from build123d import *

# Parameters (mm, degrees)
BASE_START                 = 0.7
TOP_PROFILE_W              = 8.7
TOP_PROFILE_H              = 4.4
BASE_DEPTH                 = 4
BASE_START_2               = -2.2
BASE_EXTRUDE_DEPTH         = 4.4
BOTTOM_START               = 2.2
FRONT_PROFILE_4_W          = 4.7
FRONT_PROFILE_4_H          = 0.65
BOTTOM_FRONT_CUTOUT_DEPTH  = 0.2
BOTTOM_START_2             = -2.2
FRONT_PROFILE_5_W          = 4.7
FRONT_PROFILE_5_H          = 0.65
BOTTOM_REAR_CUTOUT_DEPTH   = 0.2
SWITCH_START               = 2.2
FRONT_PROFILE_6_W          = 4.15
FRONT_PROFILE_6_H          = 2.1
FRONT_PROFILE_6_W_2        = 2
FRONT_PROFILE_6_H_2        = 2
SWITCH_INSET_DEPTH         = 0.2
UNDERCUT_NOTCH_DEPTH       = 7.771447408
UNDERCUT_NOTCH_DEPTH_BACK  = 7.771447408
LEVER_DEPTH                = 8
LEVER_DEPTH_BACK           = 2.2
LEVER_START                = 2.2
FRONT_PROFILE_7_W          = 2
FRONT_PROFILE_7_H          = 2
RIGHT_START                = 3.95
RIGHT_PIN_DEPTH            = 0.4
LEFT_START                 = -4.35
LEFT_PIN_DEPTH             = 0.4
ELECTRICAL_PINS_DEPTH      = 4.7
ELECTRICAL_PINS_DEPTH_BACK = 2.6
PINS_R                     = 0.25
LEVER_NOTCH_DEPTH          = 13.043774325
LEVER_NOTCH_DEPTH_BACK     = 13.043774325
TOP_FILLET_R               = 0.25
PIN_FILLET_R               = 0.25


with BuildPart() as part:
    # Top Profile → Base (new body)
    with BuildSketch(Plane(origin=(0, 0, 0), x_dir=(1, 0, 0), z_dir=(0, 1, 0)).offset(BASE_START)):
        Rectangle(TOP_PROFILE_W, TOP_PROFILE_H)
    extrude(amount=BASE_DEPTH)

    # Front Profile → Base Extrude (add)
    with BuildSketch(Plane.XY.offset(BASE_START_2)):
        with BuildLine():
            Line((4.35, 0.7), (4.35, 4.7))
            Line((4.35, 4.7), (-4.35, 4.7))
            Line((-4.35, 4.7), (-4.35, 0.7))
            Line((-4.35, 0.7), (-3.35, 0.7))
            Line((-3.35, 0.7), (-3.35, 0.25))
            ThreePointArc((-3.35, 0.25), (-3.276776695, 0.073223305), (-3.1, 0))
            Line((-3.1, 0), (-2.6, 0))
            ThreePointArc((-2.6, 0), (-2.423223305, 0.073223305), (-2.35, 0.25))
            Line((-2.35, 0.25), (-2.35, 0.7))
            Line((-2.35, 0.7), (-2.35, 1.35))
            Line((-2.35, 1.35), (2.35, 1.35))
            Line((2.35, 1.35), (2.35, 0.7))
            Line((2.35, 0.7), (2.35, 0.25))
            ThreePointArc((2.35, 0.25), (2.423223305, 0.073223305), (2.6, 0))
            Line((2.6, 0), (3.1, 0))
            ThreePointArc((3.1, 0), (3.276776695, 0.073223305), (3.35, 0.25))
            Line((3.35, 0.25), (3.35, 0.7))
            Line((3.35, 0.7), (4.35, 0.7))
        make_face()
    extrude(amount=BASE_EXTRUDE_DEPTH)

    # Front Profile<4> → Bottom Front Cutout (cut)
    with BuildSketch(Plane.XY.offset(BOTTOM_START)):
        with Locations((0, 1.025)):
            Rectangle(FRONT_PROFILE_4_W, FRONT_PROFILE_4_H)
    extrude(amount=-BOTTOM_FRONT_CUTOUT_DEPTH, mode=Mode.SUBTRACT)

    # Front Profile<5> → Bottom Rear Cutout (cut)
    with BuildSketch(Plane.XY.offset(BOTTOM_START_2)):
        with Locations((0, 1.025)):
            Rectangle(FRONT_PROFILE_5_W, FRONT_PROFILE_5_H)
    extrude(amount=BOTTOM_REAR_CUTOUT_DEPTH, mode=Mode.SUBTRACT)

    # Front Profile<6> → Switch Inset (cut)
    # profile 1 of 2: a face of its own
    with BuildSketch(Plane.XY.offset(SWITCH_START)):
        with Locations((0, 2.55)):
            Rectangle(FRONT_PROFILE_6_W, FRONT_PROFILE_6_H)
        with Locations((-1, 2.55)):
            Rectangle(FRONT_PROFILE_6_W_2, FRONT_PROFILE_6_H_2, mode=Mode.SUBTRACT)
    # profile 2 of 2: a face of its own
    with BuildSketch(Plane.XY.offset(SWITCH_START)):
        with Locations((-1, 2.55)):
            Rectangle(FRONT_PROFILE_6_W_2, FRONT_PROFILE_6_H_2)
    extrude(amount=-SWITCH_INSET_DEPTH, mode=Mode.SUBTRACT)

    # Side Profile → Undercut Notch (cut, two sides: drawn at the far end of the back side and taken through both)
    with BuildSketch(Plane(origin=(0, 0, 0), x_dir=(0, 0, -1), z_dir=(1, 0, 0)).offset(-UNDERCUT_NOTCH_DEPTH_BACK)):
        with BuildLine():
            ThreePointArc((-1.2, 0), (-0.8, 0.4), (-0.4, 0))
            Line((-0.4, 0), (-1.2, 0))
        make_face()
        with BuildLine():
            ThreePointArc((0.4, 0), (0.8, 0.4), (1.2, 0))
            Line((1.2, 0), (0.4, 0))
        make_face()
        with BuildLine():
            ThreePointArc((-0.8, 0.4), (-0.517157288, 0.282842712), (-0.4, 0))
            Line((-0.4, 0), (0.4, 0))
            ThreePointArc((0.4, 0), (0.517157288, 0.282842712), (0.8, 0.4))
            Line((0.8, 0.4), (-0.8, 0.4))
        make_face()
    extrude(amount=UNDERCUT_NOTCH_DEPTH + UNDERCUT_NOTCH_DEPTH_BACK, mode=Mode.SUBTRACT)

    # Front Profile<7> → Lever (add, two sides: drawn at the far end of the back side and taken through both)
    with BuildSketch(Plane.XY.offset(LEVER_START - LEVER_DEPTH_BACK)):
        with Locations((-1, 2.55)):
            Rectangle(FRONT_PROFILE_7_W, FRONT_PROFILE_7_H)
    extrude(amount=LEVER_DEPTH + LEVER_DEPTH_BACK)

    # Side Profile<5> → Right Pin (add)
    with BuildSketch(Plane(origin=(0, 0, 0), x_dir=(0, 0, -1), z_dir=(1, 0, 0)).offset(RIGHT_START)):
        Polygon((-0.4, 0), (0.4, 0), (0.6, -1.25), (0.15, -2.5), (-0.15, -2.5), (-0.6, -1.25), align=None)
        with BuildLine():
            ThreePointArc((-0.8, 0.4), (-0.517157288, 0.282842712), (-0.4, 0))
            Line((-0.4, 0), (0.4, 0))
            ThreePointArc((0.4, 0), (0.517157288, 0.282842712), (0.8, 0.4))
            Line((0.8, 0.4), (-0.8, 0.4))
        make_face()
        with BuildLine():
            Line((2.2, 4.7), (-2.2, 4.7))
            Line((-2.2, 4.7), (-2.2, 0.7))
            Line((-2.2, 0.7), (-2.2, 0))
            Line((-2.2, 0), (-1.2, 0))
            ThreePointArc((-1.2, 0), (-1.082842712, 0.282842712), (-0.8, 0.4))
            Line((-0.8, 0.4), (0.8, 0.4))
            ThreePointArc((0.8, 0.4), (1.082842712, 0.282842712), (1.2, 0))
            Line((1.2, 0), (2.2, 0))
            Line((2.2, 0), (2.2, 0.7))
            Line((2.2, 0.7), (2.2, 4.7))
        make_face()
    extrude(amount=RIGHT_PIN_DEPTH)

    # Side Profile<6> → Left Pin (add)
    with BuildSketch(Plane(origin=(0, 0, 0), x_dir=(0, 0, -1), z_dir=(1, 0, 0)).offset(LEFT_START)):
        Polygon((-0.4, 0), (0.4, 0), (0.6, -1.25), (0.15, -2.5), (-0.15, -2.5), (-0.6, -1.25), align=None)
        with BuildLine():
            ThreePointArc((-0.8, 0.4), (-0.517157288, 0.282842712), (-0.4, 0))
            Line((-0.4, 0), (0.4, 0))
            ThreePointArc((0.4, 0), (0.517157288, 0.282842712), (0.8, 0.4))
            Line((0.8, 0.4), (-0.8, 0.4))
        make_face()
        with BuildLine():
            Line((2.2, 4.7), (-2.2, 4.7))
            Line((-2.2, 4.7), (-2.2, 0.7))
            Line((-2.2, 0.7), (-2.2, 0))
            Line((-2.2, 0), (-1.2, 0))
            ThreePointArc((-1.2, 0), (-1.082842712, 0.282842712), (-0.8, 0.4))
            Line((-0.8, 0.4), (0.8, 0.4))
            ThreePointArc((0.8, 0.4), (1.082842712, 0.282842712), (1.2, 0))
            Line((1.2, 0), (2.2, 0))
            Line((2.2, 0), (2.2, 0.7))
            Line((2.2, 0.7), (2.2, 4.7))
        make_face()
    extrude(amount=LEFT_PIN_DEPTH)

    # Pins → Electrical Pins (add, two sides: drawn at the far end of the back side and taken through both)
    with BuildSketch(Plane(origin=(0, 0, 0), x_dir=(1, 0, 0), z_dir=(0, 1, 0)).offset(-ELECTRICAL_PINS_DEPTH_BACK)):
        with Locations(Location((-2, 0, 0), (0, 0, 270))):
            Circle(PINS_R)
        with Locations(Location((0, 0, 0), (0, 0, 270))):
            Circle(PINS_R)
        with Locations(Location((2, 0, 0), (0, 0, 270))):
            Circle(PINS_R)
    extrude(amount=ELECTRICAL_PINS_DEPTH + ELECTRICAL_PINS_DEPTH_BACK)

    # Lever Notch Profile → Lever Notch (cut, two sides: drawn at the far end of the back side and taken through both)
    with BuildSketch(Plane(origin=(0, 0, 0), x_dir=(1, 0, 0), z_dir=(0, 1, 0)).offset(-LEVER_NOTCH_DEPTH_BACK)):
        Polygon((-1.5, -10.2), (-0.5, -10.2), (-1, -9.7), align=None)
    extrude(amount=LEVER_NOTCH_DEPTH + LEVER_NOTCH_DEPTH_BACK, mode=Mode.SUBTRACT)

    # Top Fillet
    top_fillet_edges = [part.edges().sort_by_distance(p)[0] for p in [
        (0, 4.7, 2.2),
        (4.35, 4.7, 0),
        (0, 4.7, -2.2),
        (-4.35, 4.7, 0),
    ]]
    fillet(top_fillet_edges, radius=TOP_FILLET_R)

    # Pin Fillet
    pin_fillet_edges = [part.edges().sort_by_distance(p)[0] for p in [
        (-2, -2.6, -0.25),
        (0, -2.6, -0.25),
        (2, -2.6, -0.25),
    ]]
    fillet(pin_fillet_edges, radius=PIN_FILLET_R)


solid = part.part
Input: part model. Units: mm. Frame: model coordinates. A direction names the side the tool comes from. Give positions to 0.01 mm unless a question says otherwise; leave off trailing zeros. Write each loop counter-clockwise with the first axis right and the second up, starting at its lowest first coordinate (ties: lowest second). Pieces come first, ordered by that corner, then holes. Notation, with made-up numbers: M 14,-20.75 L 56,-20.75 A7 cw 56,-11.75 Z; hole C 0.25,-28.5 d5. An arc over 180 degrees is marked long. Write item = value, one per line. Start each with the question number.
1) Cut plane B-B on y = 1.75. Return the cut outline in (x, z) (3 decimals).
2) Draft query along Z for faces 1 (the flat face through (-3, 0.4, 0)), 2 (the flat face through (-3.95, 0, 0)), 3 (the flat face through (0, 3, -2.2)). Return one class per face: +Z half, -Z half, draft (parallel to the pull), parting line (faces both ways), or undercut.
3) First-contact query: pin 1 Ø0.6 at (y, z) = (2.5, 7) entering from +X; pin 2 Ø2 at (x, z) = (-0.5, 5.5) entering from +Y; pin 3 Ø2 at (x, y) = (-3, -0.5) entering from -Z; pin 4 Ø1.3 at (x, y) = (1.5, 3.5) entering from +Z. Flat tips, straight axial feed; report the tip coordinate or a pass-through.
4) Cut plane A-A on x = 0.75. Return the cut outline in (y, z), then the cut area to 3 significant figures.
5) Cut plane D-D on z = 7. Return the cut outline in (x, y), then the cut area to 3 significant figures.
6) Reachability of faces 4 (the flat face through (3, 0.4, 0)), 5 (the flat face through (0, 4.7, 0)), 6 (the flat face through (3.95, 0, 0)) from +Z, -Z, +X, -X, +Y, -Y: full face, straight path, thin tool, end or side. Return the list, or none.
7) Material intervals for line 1 along X through (y, z) = (-0.25, 0); line 2 along Y through (x, z) = (-1, -0.5); line 3 along X through (y, z) = (2.75, 7.5), sorted ascending. Write a range as [from, to].
Solved:
q1.outline = M -4.35,-2.2 L 4.35,-2.2 L 4.35,2.2 L 2.075,2.2 L 2.075,2 L 0,2 L 0,10.2 L -0.5,10.2 L -1,9.7 L -1.5,10.2 L -2,10.2 L -2,2 L -2.075,2 L -2.075,2.2 L -4.35,2.2 Z
q2.face_1 = undercut
q2.face_2 = draft
q2.face_3 = -Z half
q3.pin_1 = 0
q3.pin_2 = 3.55
q3.pin_3 = -2.2
q3.pin_4 = 2.2
q4.outline = M 0.7,-2 L 1.35,-2 L 1.35,-2.2 L 4.45,-2.2 A0.25 ccw 4.7,-1.95 L 4.7,1.95 A0.25 ccw 4.45,2.2 L 3.6,2.2 L 3.6,2 L 1.5,2 L 1.5,2.2 L 1.35,2.2 L 1.35,2 L 0.7,2 Z
q4.area = 16.9 mm2
q5.outline = M -2,1.55 L 0,1.55 L 0,3.55 L -2,3.55 Z
q5.area = 4.00 mm2
q6.face_4 = -Y
q6.face_5 = +Z, -Z, +X, -X, +Y
q6.face_6 = +Z, -Z, -Y
q7.line_1 = [-4.35, -3.95], [-2.25, -1.75], [-0.25, 0.25], [1.75, 2.25], [3.95, 4.35]
q7.line_2 = [0.7, 4.7]
q7.line_3 = [-2, 0]
